Geometry check sheet. Reference: the model listing, model coordinates, mm. Face numbers are marked on the shaded views. A direction names the side the tool comes from. Coordinates: 2 decimals unless noted, no trailing zeros. Order: outer loops, then holes, each group sorted by start corner. A loop starts at its lowest first (then second) coordinate and runs counter-clockwise, first axis right, second up. Notation, with made-up numbers: (70, 51.25) - (128, 51.25) arc R19 cw to (128, 70.25) - close; hole circle Ø10 at (80, 27). An arc over 180 degrees is marked (long way). Use CSV: the item, a comma, the result in double quotes. Start each with the question number.
1) Sectioned sample at A-A, the plane x = 7. Record the cut outline in (y, z), and give its area (3 significant figures).
2) Sectioned sample at C-C, the plane x = 13.5. Record the cut outline in (y, z).
3) Tool access check on the marked faces 1, 2 and 3. Record the directions out of +Z, -Z, +X, -X, +Y, -Y that give a thin tool (end or side, any length) a straight path to the whole face; none if there is none.
4) Depth check by flat-ended pin: P1, Ø2, axis at y = 10, z = 2, coming from the +X side; P2, Ø3, axis at y = 25.5, z = 5, coming from the +X side; P3, Ø1.6, axis at x = 8.87, y = 32.21, coming from the -Z side. Enter the tip coordinate at first touch or a pass-through.
5) Thickness scan on probe 1 along Z at (x, y) = (10, 31.5); probe 2 along Y at (x, z) = (-1, 10.5); probe 3 along Y at (x, z) = (1.5, 1.75). Record the ranges inside material, lowest first. Write a range as [from, to].
6) Draft check along Y on the marked faces 4, 5, 6 and 7. Enter one of: released by +Y, released by -Y, zero draft, split by the parting line, or undercut.
7) Sectioned sample at B-B, the plane y = 22. Record the cut outline in (x, z).
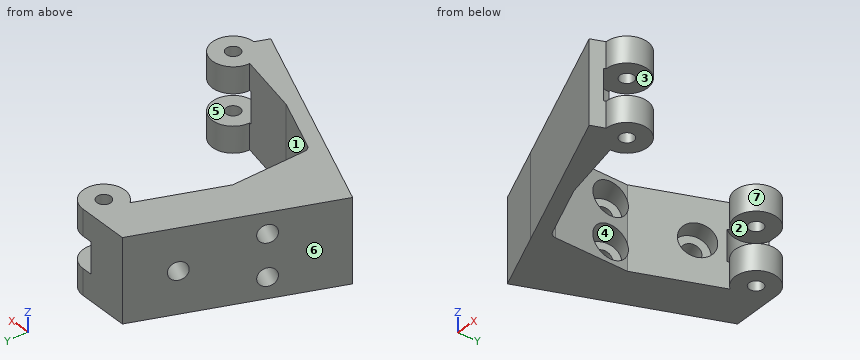
from build123d import *

# Parameters (mm, degrees)
SKETCH1_R                     = 1
BOSS_EXTRUDE1_DEPTH           = 12
SKETCH2_R                     = 3.3
CUT_EXTRUDE1_DEPTH            = 2.25
CUT_EXTRUDE1_DEPTH_BACK       = 2.25
FILLET3_R                     = 1
BOSS_EXTRUDE2_REACH           = 51.61
SKETCH4_W                     = 12
SKETCH4_H                     = 26.489515253
HOLE_SKETCH_R                 = 1.288405797
SCREW_SHAFT_HOLES_DEPTH       = 42.118659034
SCREW_SHAFT_HOLES_DEPTH_BACK  = 42.118659034
SKETCH5_R                     = 2.38125
SCREW_COUNTERBORES_DEPTH      = 5
SCREW_COUNTERBORES_DEPTH_BACK = 2.591836735
SKETCH6_W                     = 18.725223932
SKETCH6_H                     = 35.053619202
CUT_EXTRUDE2_DEPTH            = 1.66


with BuildPart() as part:
    # Sketch1 → Boss-Extrude1 (new body)
    with BuildSketch(Plane.XY):
        with BuildLine():
            Line((0, 6.640670196), (0, 35.210532713))
            Line((0, 35.210532713), (8.865440207, 35.210532713))
            ThreePointArc((8.865440207, 35.210532713), (11.575609349, 30.924071201), (6.541088012, 30.31385486))
            Line((6.541088012, 30.31385486), (2, 19.07426762))
            Line((2, 19.07426762), (2, 7.989687229))
            Line((2, 7.989687229), (10.406938735, 4.593063501))
            Line((10.406938735, 4.593063501), (19.199232805, 2.828667434))
            ThreePointArc((19.199232805, 2.828667434), (24.320553148, 4.949987778), (22.199232805, -0.171332566))
            Line((22.199232805, -0.171332566), (21.450019618, -2.025700275))
            Line((21.450019618, -2.025700275), (0, 6.640670196))
        make_face()
        with Locations((8.865440207, 32.210532713)):
            Circle(SKETCH1_R, mode=Mode.SUBTRACT)
        with Locations((22.199232805, 2.828667434)):
            Circle(SKETCH1_R, mode=Mode.SUBTRACT)
    extrude(amount=BOSS_EXTRUDE1_DEPTH)

    # Sketch2 → Cut-Extrude1 (cut, two sides)
    with BuildSketch(Plane.XY.offset(6)) as cut_extrude1_sk:
        with Locations((8.865440207, 32.210532713)):
            Circle(SKETCH2_R)
        with Locations((22.199232805, 2.828667434)):
            Circle(SKETCH2_R)
    extrude(amount=CUT_EXTRUDE1_DEPTH, mode=Mode.SUBTRACT)
    extrude(cut_extrude1_sk.sketch, amount=-CUT_EXTRUDE1_DEPTH_BACK, mode=Mode.SUBTRACT)

    # Fillet3
    fillet3_edges = [part.edges().sort_by_distance(p)[0] for p in [
        (2, 7.989687229, 6),
    ]]
    fillet(fillet3_edges, radius=FILLET3_R)

    # Boss-Extrude2: up to this face of the body (flat: up to its plane)
    boss_extrude2_end = Plane(part.part.faces().sort_by_distance((0, 20.925601454, 6))[0])
    # Sketch4 → Boss-Extrude2 (add, up to the picked face)
    with BuildSketch(Plane(origin=(-12.229645639, 4.941097571, 0), x_dir=(0, 0, -1), z_dir=(-0.9271838545667871, 0.37460659341591285, 0)), mode=Mode.PRIVATE) as boss_extrude2_sk1:
        with Locations((-6, -19.401879815)):
            Rectangle(SKETCH4_W, SKETCH4_H)
    boss_extrude2_tool1 = split(extrude(boss_extrude2_sk1.sketch, amount=-BOSS_EXTRUDE2_REACH, mode=Mode.PRIVATE), bisect_by=boss_extrude2_end, keep=Keep.BOTH, mode=Mode.PRIVATE)
    add(boss_extrude2_tool1.solids().sort_by(Axis((-4.961574, 22.930207, 6), (0.9271838545667871, -0.37460659341591285, 0)))[0])

    # Hole sketch → Screw shaft holes (cut, two sides)
    with BuildSketch(Plane(origin=(7.68361222, 33.141701506, 0), x_dir=(0, 0, -1), z_dir=(-0.927183854566786, 0.3746065934159158, 0))) as screw_shaft_holes_sk:
        with Locations(Location((-9, 17.420162392, 0), (0, 0, 270))):
            Circle(HOLE_SKETCH_R)
        with Locations(Location((-3, 17.420162392, 0), (0, 0, 270))):
            Circle(HOLE_SKETCH_R)
        with Locations(Location((-6, 6.887654186, 0), (0, 0, 90))):
            Circle(HOLE_SKETCH_R)
    extrude(amount=SCREW_SHAFT_HOLES_DEPTH, mode=Mode.SUBTRACT)
    extrude(screw_shaft_holes_sk.sketch, amount=-SCREW_SHAFT_HOLES_DEPTH_BACK, mode=Mode.SUBTRACT)

    # Sketch5 → Screw counterbores (cut, two sides)
    with BuildSketch(Plane(origin=(-4.905710031, 1.982035509, 0), x_dir=(0, 0, -1), z_dir=(0.927183854566786, -0.3746065934159158, 0))) as screw_counterbores_sk:
        with Locations(Location((-6, 26.719128162, 0), (0, 0, 270))):
            Circle(SKETCH5_R)
        with Locations(Location((-9, 16.186619957, 0), (0, 0, 109.262094827))):
            Circle(SKETCH5_R)
        with Locations(Location((-3, 16.186619957, 0), (0, 0, 109.262094827))):
            Circle(SKETCH5_R)
    extrude(amount=SCREW_COUNTERBORES_DEPTH, mode=Mode.SUBTRACT)
    extrude(screw_counterbores_sk.sketch, amount=-SCREW_COUNTERBORES_DEPTH_BACK, mode=Mode.SUBTRACT)

    # Sketch6 → Cut-Extrude2 (cut)
    with BuildSketch(Plane(origin=(-12.229645639, 4.941097571, 0), x_dir=(0, 0, 1), z_dir=(-0.9271838545667871, 0.37460659341591296, 0))):
        with Locations((5.962549552, 20.221942298)):
            Rectangle(SKETCH6_W, SKETCH6_H)
    extrude(amount=-CUT_EXTRUDE2_DEPTH, mode=Mode.SUBTRACT)


solid = part.part
Evaluation:
1,outline,"(3.81, 0) - (5.97, 0) - (5.97, 12) - (3.81, 12) - close; (29.86, 0) - (35.21, 0) - (35.21, 12) - (29.86, 12) - (29.86, 8.25) - (34.93, 8.25) - (34.93, 3.75) - (29.86, 3.75) - close"
1,area,"67.3 mm²"
2,outline,"(1.19, 0) - (3.97, 0) - (3.97, 12) - (1.19, 12) - close"
3,face 1,"+Z, -Z"
3,face 2,"+X"
3,face 3,"+X, +Y"
4,P1,"x = 2"
4,P2,"x = 4.89"
4,P3,"through"
5,probe 1,"[0, 3.75], [8.25, 12]"
5,probe 2,"[7.04, 15.87], [18.57, 28.3]"
5,probe 3,"[6.03, 14.67], [19.04, 34.49]"
6,face 4,"undercut"
6,face 5,"zero draft"
6,face 6,"released by +Y"
6,face 7,"undercut"
7,outline,"(-3.55, 0) - (3.18, 0) - (3.18, 12) - (-3.55, 12) - close"
